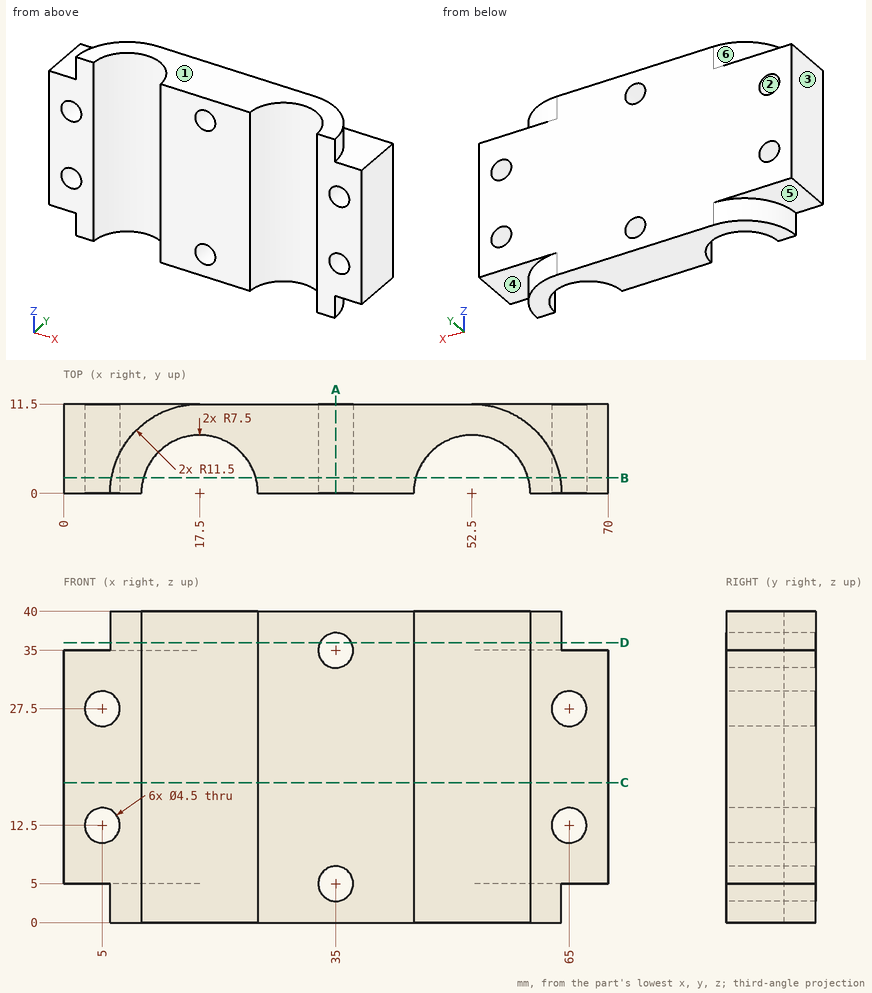
The drawing under review shows one solid part. Ordinate dimensions are in mm from its lowest x, y, z. A direction names the side the tool comes from. Round coordinates to 2 decimals unless told otherwise and drop trailing zeros. Loops run counter-clockwise (first coordinate to the right, second up) from the corner with the lowest first, then second, coordinate; pieces in that order, holes last. Notation, with made-up numbers: (71.25, 75.25) -> (106.25, 75.25) arc R30 cw to (106.25, 102.25) -> close; hole circle Ø3 at (-9.75, 21). An arc over 180 degrees is marked (long way). One line per question, with ' | ' between items. Start each with the question number.
Item 1: Wall thickness on line 1 along X through (y, z) = (8.5, 12.5); line 2 along Z through (x, y) = (65, 7); line 3 along Z through (x, y) = (35, 5.5): over which ranges is each line inside the solid? List them lowest first. Write a range as [from, to].
Item 2: Machinability: for the marked faces 4, 5 and 6, which of the approach directions +Z, -Z, +X, -X, +Y, -Y give a long, thin tool a straight path to every point of the face, cutting with its end or side? Answer none if there is none.
Item 3: Add section D-D, the plane z = 36. Write out the cut boundary in (x, y), then the cut area to 3 significant figures.
Item 4: Draft analysis for pull direction X (two halves, no side actions). For the marked faces 1, 2 and 3, state which applies: +X half, -X half, draft (parallel to the pull), parting line (faces both ways), or undercut.
Item 5: Add section A-A, the plane x = 35. Write out the cut boundary in (y, z), then the cut area to 4 significant figures.
Item 6: Add section C-C, the plane z = 18. Write out the cut boundary in (x, y), then the cut area to 3 significant figures.
Item 7: For pin 1 (1 mm diameter, centred on x = 16, z = 20, fed in from -Y); pin 2 (2 mm diameter, centred on x = 21.5, z = 10, fed in from -Y); pin 3 (2.5 mm diameter, centred on x = 65, z = 27.5, fed in from +Y), all flat-tipped, find the tip position at first contact; note any pin that passes through.
Item 8: Add section B-B, the plane y = 2. Count the separate pieces of the cut face and the enclosed holes in it, then the cut area to 3 significant figures.
Return value:
1) line 1: x = [0, 2.75], [7.25, 62.75], [67.25, 70] | line 2: z = [5, 10.25], [14.75, 25.25], [29.75, 35] | line 3: z = [0, 2.75], [7.25, 32.75], [37.25, 40]
2) face 4: -Z, +X, +Y | face 5: -Z, -X, +Y | face 6: +Z, -X, +Y
3) outline: (6, 0) -> (10, 0) arc R7.5 cw to (25, 0) -> (32.98, 0) -> (32.98, 11.5) -> (17.5, 11.5) arc R11.5 ccw to start; (37.02, 0) -> (45, 0) arc R7.5 cw to (60, 0) -> (64, 0) arc R11.5 ccw to (52.5, 11.5) -> (37.02, 11.5) -> close | area: 387 mm2
4) face 1: draft | face 2: undercut | face 3: -X half
5) outline: (0, 0) -> (11.5, 0) -> (11.5, 2.75) -> (0, 2.75) -> close; (0, 7.25) -> (11.5, 7.25) -> (11.5, 32.75) -> (0, 32.75) -> close; (0, 37.25) -> (11.5, 37.25) -> (11.5, 40) -> (0, 40) -> close | area: 356.5 mm2
6) outline: (0, 0) -> (10, 0) arc R7.5 cw to (25, 0) -> (45, 0) arc R7.5 cw to (60, 0) -> (70, 0) -> (70, 11.5) -> (0, 11.5) -> close | area: 628 mm2
7) pin 1: stops at y = 7.23 | pin 2: stops at y = 5.59 | pin 3: passes through
8) separate pieces: 3 | enclosed holes: 6 | area: 1,420 mm2
